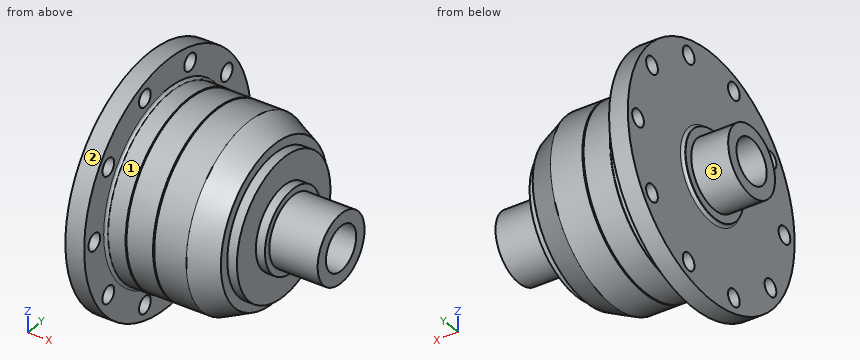
from build123d import *

# Parameters (mm, degrees)
SKETCH2_R      = 5
EXTRUDE1_DEPTH = 10.95
FILLET3_R      = 1.5


with BuildPart() as part:
    # Sketch1 → Revolve1 (revolve)
    with BuildSketch(Plane.XY):
        Polygon((0, 53), (0, 71.2), (-10.95, 71.2), (-10.95, 42.087444297), (-10.95, 24.85), (-12.95, 24.85), (-12.95, 20), (-34.5, 20), (-34.5, 12.9), (101.3, 12.9), (101.3, 20), (73.1, 20), (73.1, 23.75), (67.8, 23.75), (67.8, 39.95), (62.2, 39.95), (62.2, 45.45), (46.9, 52.7), (28.240404552, 52.7), (28.240404552, 51.349259098), (27.559120448, 51.349259098), (27.559120448, 52.7), (12.131909835, 52.7), (12.131909835, 50.122589957), (11.761037764, 50.122589957), (11.761037764, 53), align=None)
    revolve(axis=Axis((-78.843245127, 0, 0), (1, 0, 0)))

    # Sketch2 → Extrude1 (cut)
    with BuildSketch(Plane.ZY.offset(10.95)):
        with Locations((0, 62.5)):
            Circle(SKETCH2_R)
        with Locations((36.736578268, 50.563562148)):
            Circle(SKETCH2_R)
        with Locations((59.441032268, 19.313562148)):
            Circle(SKETCH2_R)
        with Locations((59.441032268, -19.313562148)):
            Circle(SKETCH2_R)
        with Locations((36.736578268, -50.563562148)):
            Circle(SKETCH2_R)
        with Locations((0, -62.5)):
            Circle(SKETCH2_R)
        with Locations((-36.736578268, -50.563562148)):
            Circle(SKETCH2_R)
        with Locations((-59.441032268, -19.313562148)):
            Circle(SKETCH2_R)
        with Locations((-59.441032268, 19.313562148)):
            Circle(SKETCH2_R)
        with Locations((-36.736578268, 50.563562148)):
            Circle(SKETCH2_R)
    extrude(amount=-EXTRUDE1_DEPTH, mode=Mode.SUBTRACT)

    # Fillet3
    fillet3_edges = [part.edges().sort_by_distance(p)[0] for p in [
        (0, -53, 0),
        (-10.95, -24.85, 0),
    ]]
    fillet(fillet3_edges, radius=FILLET3_R)


solid = part.part
Input: part model. Units: mm. Frame: model coordinates. Face numbers are marked on the shaded views. A direction names the side the tool comes from. Coordinates: 2 decimals unless noted, no trailing zeros. Loops run counter-clockwise (first coordinate to the right, second up) from the corner with the lowest first, then second, coordinate; pieces in that order, holes last. Notation, with made-up numbers: (61.25, 4) - (86.25, 4) arc R19 ccw to (86.25, 40) - close; hole circle Ø9 at (69.5, 58.25). An arc over 180 degrees is marked (long way). Answer in a Markdown table with one row per item. Add a question column.
Item 1: Section query A-A on z = 61. Return the cut outline in (x, y).
Item 2: Section query C-C on z = 0. State how many separate pieces and enclosed holes the cut face has, then the cut area to 3 significant figures.
Item 3: Access query for the marked faces 1, 2 and 3. Directions: +Z, -Z, +X, -X, +Y, -Y. A direction counts if a zero-diameter tool reaches every point of the face in a straight line with its end or side. Return the directions, or none.
Item 4: Section query B-B on y = 62.5. Return the cut outline in (x, z).
Item 5: Line query: line 1 along X through (y, z) = (36.5, -45); line 2 along Y through (x, z) = (53, -20); line 3 along X through (y, z) = (27, 20). Output: solid intervals per line, ascending. Write a range as [from, to].
Item 6: Contact query for flat-ended pins moving along their axis: P1, Ø1, axis at y = -44.5, z = -29, coming from the -X side; P2, Ø8, axis at y = -50.56, z = -36.74, coming from the +X side; P3, Ø1.5, axis at x = 16.5, y = 22.5, coming from the +Z side; P4, Ø11.5, axis at y = 19.31, z = -59.44, coming from the -X side. Output: stop coordinate, or through.
Item 7: Section query D-D on x = 20.5. Return the cut outline in (y, z), then the cut area to 3 significant figures.
Recorded:
| question | item | result |
|---|---|---|
| 1 | outline | (-10.95, -36.72) - (0, -36.72) - (0, -24.06) - (-10.95, -24.06) - close; (-10.95, -14.56) - (0, -14.56) - (0, 14.56) - (-10.95, 14.56) - close; (-10.95, 24.06) - (0, 24.06) - (0, 36.72) - (-10.95, 36.72) - close |
| 2 | separate pieces | 4 |
| 2 | enclosed holes | 0 |
| 2 | area | 7,080 mm^2 |
| 3 | face 1 | +X |
| 3 | face 2 | +X, -X |
| 3 | face 3 | -X |
| 4 | outline | (-10.95, -34.11) - (0, -34.11) - (0, -5) - (-10.95, -5) - close; (-10.95, 5) - (0, 5) - (0, 34.11) - (-10.95, 34.11) - close |
| 5 | line 1 | [-10.95, 0] |
| 5 | line 2 | [-45.62, 45.62] |
| 5 | line 3 | [-10.95, 67.8] |
| 6 | P1 | x = -10.95 |
| 6 | P2 | through |
| 6 | P3 | z = 48 |
| 6 | P4 | x = -10.95 |
| 7 | outline | circle Ø105.4 at (0, 0); hole circle Ø25.8 at (0, 0) |
| 7 | area | 8,200 mm^2 |
